Design review of the part built by this model. Coordinates are the model's own, in mm. A direction names the side the tool comes from. Coordinates: 2 decimals unless noted, no trailing zeros. Order: outer loops, then holes, each group sorted by start corner. A loop starts at its lowest first (then second) coordinate and runs counter-clockwise, first axis right, second up. Notation, with made-up numbers: M -17,20.5 L 36,20.5 A17 cw 36,44.5 Z; hole C -30.5,4.5 d7. An arc over 180 degrees is marked long. Answer in a Markdown table with one row per item.
from build123d import *

# Parameters (mm, degrees)
ESQUISSE1_R        = 10
BOSS_EXTRU_1_DEPTH = 120
ESQUISSE2_R        = 8
BOSS_EXTRU_2_DEPTH = 10
BOSS_EXTRU_3_START = 10
ESQUISSE3_R        = 8
BOSS_EXTRU_3_DEPTH = 10


with BuildPart() as part:
    # Esquisse1 → Boss.-Extru.1 (new body)
    with BuildSketch(Plane(origin=(0, 0, 0), x_dir=(1, 0, 0), z_dir=(0, 1, 0))):
        with Locations(Location((0, 0, 0), (0, 0, 270))):
            Circle(ESQUISSE1_R)
    extrude(amount=BOSS_EXTRU_1_DEPTH)

    # Esquisse2 → Boss.-Extru.2 (add)
    with BuildSketch(Plane.XZ):
        with Locations(Location((0, 0, 0), (0, 0, 270))):
            Circle(ESQUISSE2_R)
    extrude(amount=BOSS_EXTRU_2_DEPTH)

    # Esquisse3 → Boss.-Extru.3 (add)
    with BuildSketch(Plane(origin=(0, 120, 0), x_dir=(1, 0, 0), z_dir=(0, 1, 0)).offset(BOSS_EXTRU_3_START)):
        with Locations(Location((0, 0, 0), (0, 0, 90))):
            Circle(ESQUISSE3_R)
    extrude(amount=-BOSS_EXTRU_3_DEPTH)


solid = part.part
(1) For line 1 along Y through (x, z) = (-7, -5); line 2 along X through (y, z) = (0.5, 6); line 3 along X through (y, z) = (26, -0.5), list the stretches that pass through material, from the lowest coordinate up. Write a range as from..to.
Return value:
| item | result |
|---|---|
| line 1 | y = 0..120 |
| line 2 | x = -8..8 |
| line 3 | x = -9.99..9.99 |
(2) Add section B-B, the plane x = -4. Give the boundary of the cut face in (y, z), and give its area (3 significant figures).
Return value:
| item | result |
|---|---|
| outline | M -10,-6.93 L 0,-6.93 L 0,-9.17 L 120,-9.17 L 120,-6.93 L 130,-6.93 L 130,6.93 L 120,6.93 L 120,9.17 L 0,9.17 L 0,6.93 L -10,6.93 Z |
| area | 2,480 mm2 |
(3) Add section C-C, the plane y = 8. Give the boundary of the cut face in (x, z), and give its area (3 significant figures).
Return value:
| item | result |
|---|---|
| outline | C 0,0 d20 |
| area | 314 mm2 |
(4) Insertion check: pin 1 Ø3 at (x, y) = (-7.5, 71.5) entering from +Z; pin 2 Ø5 at (y, z) = (28, 3) entering from -X; pin 3 Ø4 at (y, z) = (34, -4) entering from +X. Each pin has a flat end and moves straight along its axis. Give the tip position at first contact, or say it passes through.
Return value:
| item | result |
|---|---|
| pin 1 | stops at z = 8 |
| pin 2 | stops at x = -9.99 |
| pin 3 | stops at x = 9.8 |
(5) Add section A-A, the plane z = 0. Give the boundary of the cut face in (x, y), and give its area (3 significant figures).
Return value:
| item | result |
|---|---|
| outline | M -10,0 L -8,0 L -8,-10 L 8,-10 L 8,0 L 10,0 L 10,120 L 8,120 L 8,130 L -8,130 L -8,120 L -10,120 Z |
| area | 2,720 mm2 |
(6) For faces 1 (the cylindrical face through (-7.81, -4.93, 1.73)), 2 (the flat face through (0, -10, 0)), 3 (the cylindrical face through (7.81, 125.07, 1.73)), list the 3-axis set-ups (+Z, -Z, +X, -X, +Y, -Y) from which the entire face can be reached by the end or side of a thin tool; tool diameter is ignored.
Return value:
| item | result |
|---|---|
| face 1 | -Y |
| face 2 | +Z, -Z, +X, -X, -Y |
| face 3 | +Y |
